Source: CAD feature listing. Evaluate the final solid. Frame: model axes, mm. Face numbers are marked on the shaded views. A direction names the side the tool comes from. Coordinates: 2 decimals unless noted, no trailing zeros. Write each loop counter-clockwise with the first axis right and the second up, starting at its lowest first coordinate (ties: lowest second). Pieces come first, ordered by that corner, then holes. Notation, with made-up numbers: (4.5, -6) - (63.5, -6) arc R29 cw to (63.5, 14) - close; hole circle Ø10 at (43, 54.5). An arc over 180 degrees is marked (long way). One line per item, written item: value.
Autodesk Inventor part; units mm, degrees
ref_plane "YZ Plane" through (0, 0, 0) normal (1, 0, 0) x (0, 1, 0)
ref_plane "XZ Plane" through (0, 0, 0) normal (0, 1, 0) x (-1, 0, 0)
ref_plane "XY Plane" through (0, 0, 0) normal (0, 0, 1) x (1, 0, 0)
sketch "Sketch1" plane through (0, 0, 0) normal (0, 1, 0) x (-1, 0, 0)
  line L0 (6.7, 0) -> (3.35, -5.8024)
  line L1 (3.35, -5.8024) -> (-3.35, -5.8024)
  line L2 (-3.35, -5.8024) -> (-6.7, 0)
  line L3 (-6.7, 0) -> (-3.35, 5.8024)
  line L4 (-3.35, 5.8024) -> (3.35, 5.8024)
  line L5 (3.35, 5.8024) -> (6.7, 0)
  point P0 (0, 0)
  dimension "d1" = 6.7
extrude "Extrusion1" add sketch "Sketch1" along normal blind 17
sketch "Sketch2" plane through (0, 17, 0) normal (0, 1, 0) x (1, 0, 0)
  circle A0 centre (0, 0) radius 1.25
  dimension "d4" = 2.5
extrude "Extrusion2" cut sketch "Sketch2" against normal blind 8
sketch "Sketch3" plane through (0, 17, 0) normal (0, 1, 0) x (1, 0, 0)
  circle A0 centre (0, 0) radius 1.5
  dimension "d10" = 3
extrude "Extrusion3" cut sketch "Sketch3" against normal blind 8
sketch "Sketch4" plane through (0, 0, 0) normal (0, -1, 0) x (1, 0, 0)
  circle A0 centre (0, 0) radius 1.575
  dimension "d14" = 3.15
extrude "Extrusion4" cut sketch "Sketch4" against normal blind 7
properties part number "BruteForceCoupler"
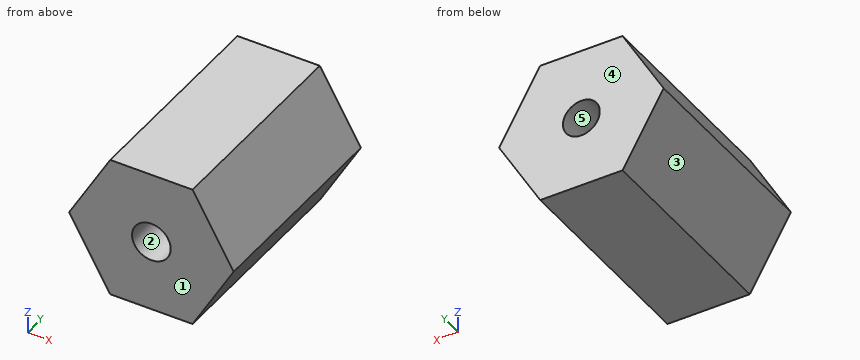
1) Reachability of the marked faces 1 and 2 from +Z, -Z, +X, -X, +Y, -Y: full face, straight path, thin tool, end or side. Return the list, or none.
Values found:
face 1: +Z, -Z, +X, -X, -Y
face 2: -Y
2) Draft query along X for the marked faces 3, 4 and 5. Return one class per face: released by +X, released by -X, zero draft, split by the parting line, or undercut.
Values found:
face 3: released by -X
face 4: zero draft
face 5: undercut
3) Section query C-C on y = 7.75. Output: boundary loops of the cut face in (x, z).
Values found:
outline: (-6.7, 0) - (-3.35, -5.8) - (3.35, -5.8) - (6.7, 0) - (3.35, 5.8) - (-3.35, 5.8) - close
4) Section query B-B on x = 0. Output: boundary loops of the cut face in (y, z) (3 decimals), then the cut area to 3 significant figures.
Values found:
outline: (0, -5.802) - (17, -5.802) - (17, -1.5) - (9, -1.5) - (9, 1.5) - (17, 1.5) - (17, 5.802) - (0, 5.802) - (0, 1.575) - (7, 1.575) - (7, -1.575) - (0, -1.575) - close
area: 151 mm2
5) Section query A-A on y = 4.75. Output: boundary loops of the cut face in (x, z) (3 decimals), then the cut area to 3 significant figures.
Values found:
outline: (-6.7, 0) - (-3.35, -5.802) - (3.35, -5.802) - (6.7, 0) - (3.35, 5.802) - (-3.35, 5.802) - close; hole circle Ø3.15 at (0, 0)
area: 109 mm2
6) Material intervals for line 1 (Z direction, x = 0, y = 13.5); line 2 (Z direction, x = 0, y = 3.5) (3 decimals); line 3 (X direction, y = 3.5, z = 2.75), sorted ascending.
Values found:
line 1: -5.8 to -1.5, 1.5 to 5.8
line 2: -5.802 to -1.575, 1.575 to 5.802
line 3: -5.11 to 5.11
7) Contact query for flat-ended pins moving along their axis: P1, Ø1.8, axis at x = 0, z = 0, coming from the +Y side; P2, Ø1.5, axis at x = -4.5, y = 5.5, coming from the -Z side; P3, Ø0.9, axis at x = 0, z = 0.5, coming from the -Y side. Output: stop coordinate, or through.
Values found:
P1: y = 9
P2: z = -5.11
P3: y = 7
8) Section query D-D on z = 0.5. Output: boundary loops of the cut face in (x, y), then the cut area to 3 significant figures.
Values found:
outline: (-6.41, 0) - (-1.49, 0) - (-1.49, 7) - (1.49, 7) - (1.49, 0) - (6.41, 0) - (6.41, 17) - (1.41, 17) - (1.41, 9) - (-1.41, 9) - (-1.41, 17) - (-6.41, 17) - close
area: 174 mm2
